from build123d import *

# Parameters (mm, degrees)
BOSS_EXTRUDE1_DEPTH = 8
SKETCH2_R           = 2
BOSS_EXTRUDE2_DEPTH = 2
SHELL1_T            = -1
BOSS_EXTRUDE3_REACH = 12
SKETCH3_R           = 2.7
SKETCH3_R_2         = 1.7


with BuildPart() as part:
    # Sketch1 → Boss-Extrude1 (new body, symmetric)
    with BuildSketch(Plane(origin=(0, 0, 0), x_dir=(0, 0, -1), z_dir=(1, 0, 0))):
        Polygon((0, 0), (0, -2), (24, -2), (24, 8), (16, 8), align=None)
    extrude(amount=BOSS_EXTRUDE1_DEPTH, both=True)

    # Sketch2 → Boss-Extrude2 (add)
    with BuildSketch(Plane(origin=(0, 8, 0), x_dir=(1, 0, 0), z_dir=(0, 1, 0))):
        with Locations((-4, 20)):
            Circle(SKETCH2_R)
        with Locations((4, 20)):
            Circle(SKETCH2_R)
    extrude(amount=BOSS_EXTRUDE2_DEPTH)

    # Shell1
    shell1_openings = [part.faces().sort_by_distance(p)[0] for p in [
        (0, -2, -12),
    ]]
    offset(amount=SHELL1_T, openings=shell1_openings, kind=Kind.INTERSECTION)

    # Sketch3 → Boss-Extrude3 (add, up to next)
    with BuildSketch(Plane(origin=(0, 0, 0), x_dir=(1, 0, 0), z_dir=(0, 1, 0)), mode=Mode.PRIVATE) as boss_extrude3_sk1:
        with Locations((0, 8)):
            Circle(SKETCH3_R)
        with Locations((0, 8)):
            Circle(SKETCH3_R_2, mode=Mode.SUBTRACT)
    boss_extrude3_tool1 = extrude(boss_extrude3_sk1.sketch, amount=BOSS_EXTRUDE3_REACH, mode=Mode.PRIVATE) - part.part
    add(boss_extrude3_tool1.solids().sort_by_distance((-2.623632, 0, -8))[0])
    # Sketch3 → Boss-Extrude3 (add, up to next)
    with BuildSketch(Plane(origin=(0, 0, 0), x_dir=(1, 0, 0), z_dir=(0, 1, 0)), mode=Mode.PRIVATE) as boss_extrude3_sk2:
        with Locations((0, 16)):
            Circle(SKETCH3_R)
        with Locations((0, 16)):
            Circle(SKETCH3_R_2, mode=Mode.SUBTRACT)
    boss_extrude3_tool2 = extrude(boss_extrude3_sk2.sketch, amount=BOSS_EXTRUDE3_REACH, mode=Mode.PRIVATE) - part.part
    add(boss_extrude3_tool2.solids().sort_by_distance((-2.623632, 0, -16))[0])


solid = part.part
Geometry: final body of the model. Coordinates: model frame, mm. A direction names the side the tool comes from. Give positions to 0.01 mm unless a question says otherwise; leave off trailing zeros. Loops run counter-clockwise (first coordinate to the right, second up) from the corner with the lowest first, then second, coordinate; pieces in that order, holes last. Notation, with made-up numbers: M 5,-6 L 21,-6 A20 ccw 21,19 Z; hole C 51.25,-13.75 d11. An arc over 180 degrees is marked long. Put each result on its own line as item: value. Start each with the question number.
1) Cut plane A-A (x = -4). Output: boundary loops of the cut face in (y, z), then the cut area to 3 significant figures.
2) Cut plane C-C (y = 8.5). Output: boundary loops of the cut face in (x, z).
3) Cut plane B-B (y = 1). Output: boundary loops of the cut face in (x, z), then the cut area to 3 significant figures.
4) Contact query for flat-ended pins moving along their axis: pin 1 (2.5 mm diameter, centred on x = 1, y = 3.5, fed in from +Z); pin 2 (9 mm diameter, centred on x = 0, z = -19, fed in from +Y); pin 3 (1.6 mm diameter, centred on x = 0.5, z = -15, fed in from -Y); pin 4 (2.5 mm diameter, centred on x = -4, z = -20, fed in from -Y). Output: stop coordinate, or through.
5) Pull-direction query (X, two-part tool) for faces 1 (the flat face through (0, 7, -20)), 2 (the flat face through (1.65, 4.09, -10.42)), 3 (the flat face through (4, 10, -20)), 4 (the flat face through (-8, 2, -14)); classes: pulls with the +X half, pulls with the -X half, needs draft (parallel to the pull), parting line crosses it, or undercut.
6) Access query for faces 5 (the flat face through (0, 3, -24)), 6 (the flat face through (7, 2, -14)). Directions: +Z, -Z, +X, -X, +Y, -Y. A direction counts if a zero-diameter tool reaches every point of the face in a straight line with its end or side. Return the directions, or none.
7) Ray query, line 1 along X through (y, z) = (4.75, -16); line 2 along Z through (x, y) = (-4, 8.35); line 3 along Z through (x, y) = (0, 2.5). Return the intervals inside material, ascending.
8) Cut plane D-D (z = -9.25). Output: boundary loops of the cut face in (x, y) (3 decimals).
Verdict:
1. outline: M -2,-24 L 8,-24 L 8,-22 L 10,-22 L 10,-18 L 8,-18 L 8,-16 L 0,0 L -2,0 L -2,-1 L -0.62,-1 L 7,-16.24 L 7,-19 L 9,-19 L 9,-21 L 7,-21 L 7,-23 L -2,-23 Z
1. area: 40.0 mm2
2. outline: C -4,-20 d4; C 4,-20 d4; hole C -4,-20 d2; hole C 4,-20 d2
3. outline: M -8,-24 L 8,-24 L 8,-2 L -8,-2 Z; C 0,-16 d5.4; C 0,-8 d5.4; hole M -7,-23 L 7,-23 L 7,-4.24 L -7,-4.24 Z; hole C 0,-16 d3.4; hole C 0,-8 d3.4
3. area: 117 mm2
4. pin 1: z = -4.5
4. pin 2: y = 10
4. pin 3: y = 0
4. pin 4: y = 7
5. face 1: undercut
5. face 2: undercut
5. face 3: needs draft
5. face 4: pulls with the -X half
6. face 5: -Z, +X, -X, +Y, -Y
6. face 6: -Y
7. line 1: -8 to -7, -2.7 to -1.7, 1.7 to 2.7, 7 to 8
7. line 2: -22 to -21, -19 to -18
7. line 3: -24 to -23, -18.7 to -17.7, -14.3 to -13.3, -10.7 to -9.7, -7.24 to -5
8. outline: M -8,-2 L -7,-2 L -7,3.507 L -2.393,3.507 L -2.393,0 L -1.152,0 L -1.152,3.507 L 1.152,3.507 L 1.152,0 L 2.393,0 L 2.393,3.507 L 7,3.507 L 7,-2 L 8,-2 L 8,4.625 L -8,4.625 Z
